```python
from build123d import *

# Parameters (mm, degrees)
BOSS_EXTRUDE2_DEPTH          = 438.15
CUT_EXTRUDE1_DEPTH           = 446.936132759
F_1_4_20_TAPPED_HOLE1_REACH  = 448.053
F_1_4_20_TAPPED_HOLE1_BORE_R = 2.5527
F_1_4_20_TAPPED_HOLE2_D      = 5.1054


with BuildPart() as part:
    # Sketch1 → Boss-Extrude2 (new body)
    with BuildSketch(Plane(origin=(0, 0, 0), x_dir=(1, 0, 0), z_dir=(0, 1, 0))):
        with BuildLine():
            Line((-66.283871769, 27.377862638), (-15.483871769, 27.377862638))
            ThreePointArc((-15.483871769, 27.377862638), (-12.080917025, 14.677862638), (-2.783871769, 5.380817382))
            Line((-2.783871769, 5.380817382), (-2.783871769, 1.977862638))
            Line((-2.783871769, 1.977862638), (-78.983871769, 1.977862638))
            Line((-78.983871769, 1.977862638), (-78.983871769, 5.380817382))
            ThreePointArc((-78.983871769, 5.380817382), (-69.686826513, 14.677862638), (-66.283871769, 27.377862638))
        make_face()
    extrude(amount=BOSS_EXTRUDE2_DEPTH)

    # Sketch6 → Cut-Extrude1 (cut, through all)
    with BuildSketch(Plane(origin=(0, 0, -27.377862638), x_dir=(-1, 0, 0), z_dir=(0, 0, -1))):
        with BuildLine():
            Line((26.596371769, 425.45), (55.171371769, 425.45))
            ThreePointArc((55.171371769, 425.45), (61.90656386, 422.660192091), (64.696371769, 415.925))
            Line((64.696371769, 415.925), (64.696371769, 22.225))
            ThreePointArc((64.696371769, 22.225), (61.90656386, 15.489807909), (55.171371769, 12.7))
            Line((55.171371769, 12.7), (26.596371769, 12.7))
            ThreePointArc((26.596371769, 12.7), (19.861179678, 15.489807909), (17.071371769, 22.225))
            Line((17.071371769, 22.225), (17.071371769, 415.925))
            ThreePointArc((17.071371769, 415.925), (19.861179678, 422.660192091), (26.596371769, 425.45))
        make_face()
    extrude(amount=-CUT_EXTRUDE1_DEPTH, mode=Mode.SUBTRACT)

    # 1/4-20 Tapped Hole1 bore → 1/4-20 Tapped Hole1 (cut, up to next)
    with BuildSketch(Plane(origin=(0, 0, 0), x_dir=(-1, 0, 0), z_dir=(0, -1, 0)), mode=Mode.PRIVATE) as f_1_4_20_tapped_hole1_sk1:
        with Locations((40.883871769, 14.677862638)):
            Circle(F_1_4_20_TAPPED_HOLE1_BORE_R)
    f_1_4_20_tapped_hole1_tool1 = extrude(f_1_4_20_tapped_hole1_sk1.sketch, amount=-F_1_4_20_TAPPED_HOLE1_REACH, mode=Mode.PRIVATE) & part.part
    # 1/4-20 Tapped Hole1 bore → 1/4-20 Tapped Hole1 (cut, up to next)
    with BuildSketch(Plane(origin=(0, 0, 0), x_dir=(-1, 0, 0), z_dir=(0, -1, 0)), mode=Mode.PRIVATE) as f_1_4_20_tapped_hole1_sk2:
        with Locations((56.758871769, 14.677862638)):
            Circle(F_1_4_20_TAPPED_HOLE1_BORE_R)
    f_1_4_20_tapped_hole1_tool2 = extrude(f_1_4_20_tapped_hole1_sk2.sketch, amount=-F_1_4_20_TAPPED_HOLE1_REACH, mode=Mode.PRIVATE) & part.part
    # 1/4-20 Tapped Hole1 bore → 1/4-20 Tapped Hole1 (cut, up to next)
    with BuildSketch(Plane(origin=(0, 0, 0), x_dir=(-1, 0, 0), z_dir=(0, -1, 0)), mode=Mode.PRIVATE) as f_1_4_20_tapped_hole1_sk3:
        with Locations((25.008871769, 14.677862638)):
            Circle(F_1_4_20_TAPPED_HOLE1_BORE_R)
    f_1_4_20_tapped_hole1_tool3 = extrude(f_1_4_20_tapped_hole1_sk3.sketch, amount=-F_1_4_20_TAPPED_HOLE1_REACH, mode=Mode.PRIVATE) & part.part
    add(f_1_4_20_tapped_hole1_tool1.solids().sort_by_distance((-40.883872, 0, -14.677863))[0], mode=Mode.SUBTRACT)
    add(f_1_4_20_tapped_hole1_tool2.solids().sort_by_distance((-56.758872, 0, -14.677863))[0], mode=Mode.SUBTRACT)
    add(f_1_4_20_tapped_hole1_tool3.solids().sort_by_distance((-25.008872, 0, -14.677863))[0], mode=Mode.SUBTRACT)

    # 1/4-20 Tapped Hole2 (through all)
    with Locations(Plane(origin=(0, 438.15, 0), x_dir=(1, 0, 0), z_dir=(0, 1, 0))):
        with Locations((-56.758871769, 14.677862638), (-40.883871769, 14.677862638), (-25.008871769, 14.677862638)):
            Hole(F_1_4_20_TAPPED_HOLE2_D / 2)


solid = part.part
```
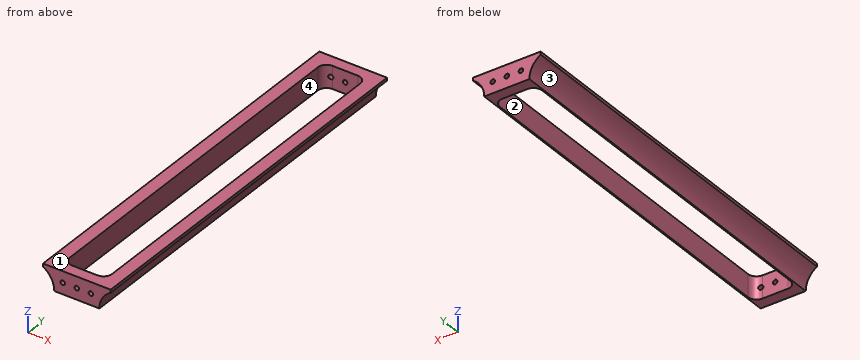
The listing builds one solid part. Answer for the finished solid, in the listing's coordinates (mm). Face numbers are marked on the shaded views. A direction names the side the tool comes from. Give positions to 0.01 mm unless a question says otherwise; leave off trailing zeros. Loops run counter-clockwise (first coordinate to the right, second up) from the corner with the lowest first, then second, coordinate; pieces in that order, holes last. Notation, with made-up numbers: (83, 42.25) - (139, 42.25) arc R25 cw to (139, 70.25) - close; hole circle Ø10 at (61, -20). An arc over 180 degrees is marked (long way). Return JSON: item names as keys, results as strings. Group by question number.
1. Straight lines are drawn through the part: line 1 (Y direction, x = -28.5, z = -6); line 2 (X direction, y = 92, z = -26); line 3 (X direction, y = 224, z = -16). For each, find the intervals that lie inside material, in ascending order. Write a range as [from, to].
2. Find section A-A (y = 398). Write down the section's boundary in (x, z).
3. Given pin 1 Ø4 at (y, z) = (188, -11) entering from +X; pin 2 Ø4.5 at (x, z) = (-56.76, -14.68) entering from -Y; pin 3 Ø1.5 at (y, z) = (253, -13) entering from -X; pin 4 Ø1 at (x, y) = (-69, 241.5) entering from -Z, each flat-ended and moving along its own axis, determine where each tip first touches the part or whether it passes through.
4. Find section B-B (x = -11.5). Write down the section's boundary in (y, z), then the cut area to 3 significant figures.
5. Find section C-C (x = -71.5). Write down the section's boundary in (y, z), then the cut area to 3 significant figures.
6. Determine the mould class of the marked faces 1 and 2 for opening direction Y: pulls with the +Y half, pulls with the -Y half, needs draft (parallel to the pull), parting line crosses it, or undercut.
7. Which of the six approach directions +Z, -Z, +X, -X, +Y, -Y give full straight-line access (tool end or side, diameter ignored) to the marked faces 3 and 4?
Verdict:
{
 "1": {"line 1": "y = [0, 12.7], [425.45, 438.15]", "line 2": "x = [-66.32, -64.7], [-17.07, -15.45]", "line 3": "x = [-68.97, -64.7], [-17.07, -12.79]"},
 "2": {"outline": "(-78.98, -5.38) arc R25.4 cw to (-66.28, -27.38) - (-64.7, -27.38) - (-64.7, -1.98) - (-78.98, -1.98) - close; (-17.07, -27.38) - (-15.48, -27.38) arc R25.4 cw to (-2.78, -5.38) - (-2.78, -1.98) - (-17.07, -1.98) - close"},
 "3": {"pin 1": "stops at x = -7.62", "pin 2": "passes through", "pin 3": "stops at x = -71.28", "pin 4": "stops at z = -17"},
 "4": {"outline": "(0, -13.72) - (438.15, -13.72) - (438.15, -1.98) - (0, -1.98) - close", "area": "5,150 mm^2"},
 "5": {"outline": "(0, -11.96) - (438.15, -11.96) - (438.15, -1.98) - (0, -1.98) - close", "area": "4,370 mm^2"},
 "6": {"face 1": "needs draft", "face 2": "undercut"},
 "7": {"face 3": "-Z, -X, +Y, -Y", "face 4": "+Z, -Z"}
}
